The model under review builds one solid part; all positions refer to its coordinate system, in mm. Face numbers are marked on the shaded views. Give positions to 0.01 mm unless a question says otherwise; leave off trailing zeros. Loops run counter-clockwise (first coordinate to the right, second up) from the corner with the lowest first, then second, coordinate; pieces in that order, holes last. Notation, with made-up numbers: (6, 5.25) - (34, 5.25) arc R20 ccw to (34, 31.25) - close; hole circle Ø5 at (-1, 68). An arc over 180 degrees is marked (long way). Return JSON: item names as keys, results as strings. Group by question number.
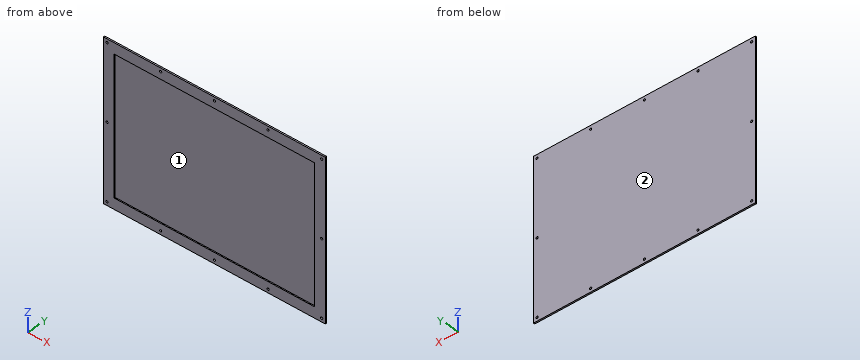
from build123d import *

# Parameters (mm, degrees)
F0_W     = 310
F0_H     = 220
F0_W_2   = 280
F0_H_2   = 190
F1_DEPTH = 2
F2_D     = 3
F3_DEPTH = 0.5


with BuildPart() as f1:
    # F0 (on Front) → F1 (new body)
    with BuildSketch(Plane.XZ):
        Rectangle(F0_W, F0_H)
        Rectangle(F0_W_2, F0_H_2, mode=Mode.SUBTRACT)
    extrude(amount=F1_DEPTH)

    # F2 (through all)
    with Locations(Plane(origin=(0, 0, 0), x_dir=(1, 0, 0), z_dir=(0, 1, 0))):
        with Locations((-150, 105), (-75, 105), (0, 105), (75, 105), (150, 105), (150, 0), (150, -105), (75, -105), (0, -105), (-75, -105), (-150, -105), (-150, 0)):
            Hole(F2_D / 2)

    # F0 (on Front) → F3 (join)
    with BuildSketch(Plane.XZ):
        Rectangle(F0_W_2, F0_H_2)
    extrude(amount=F3_DEPTH)


solid = f1.part
Item 1: Take a section at B-B (x = -36). State the section outline as (y, z) points, then the cut area to 3 significant figures.
Item 2: Mouldability with a two-part tool opening along Z and no side actions: class the marked faces 1 and 2 as +Z half, -Z half, draft (parallel to the pull), parting line (faces both ways), or undercut.
Item 3: For P1, Ø1.8, axis at x = -150, z = -105, coming from the -Y side; P2, Ø8, axis at x = 10.5, z = -80.5, coming from the -Y side, all flat-tipped, find the tip position at first contact; note any pin that passes through.
Item 4: Take a section at A-A (y = -1.4). State how many separate pieces and enclosed holes the cut face has, then the cut area to 3 significant figures.
Item 5: Take a section at C-C (z = -46). State the section outline as (x, y) points.
Item 6: For L1, parallel to X at y = -1.2, z = -105; L2, parallel to Z at x = -150, y = -0.4; L3, parallel to Z at x = 75, y = -1.25, list the stretches that pass through material, from the lowest coordinate up. Write a range as from..to.
Check sheet entries:
{
 "1": {"outline": "(-2, -110) - (0, -110) - (0, 110) - (-2, 110) - (-2, 95) - (-0.5, 95) - (-0.5, -95) - (-2, -95) - close", "area": "155 mm^2"},
 "2": {"face 1": "undercut", "face 2": "draft"},
 "3": {"P1": "passes through", "P2": "stops at y = -0.5"},
 "4": {"separate pieces": "1", "enclosed holes": "13", "area": "14,900 mm^2"},
 "5": {"outline": "(-155, -2) - (-140, -2) - (-140, -0.5) - (140, -0.5) - (140, -2) - (155, -2) - (155, 0) - (-155, 0) - close"},
 "6": {"L1": "x = -155..-151.5, -148.5..-76.5, -73.5..-1.5, 1.5..73.5, 76.5..148.5, 151.5..155", "L2": "z = -110..-106.5, -103.5..-1.5, 1.5..103.5, 106.5..110", "L3": "z = -110..-106.5, -103.5..-95, 95..103.5, 106.5..110"}
}
